Part model, mm, in its own coordinate system. Coordinates: 2 decimals unless noted, no trailing zeros. Loops run counter-clockwise (first coordinate to the right, second up) from the corner with the lowest first, then second, coordinate; pieces in that order, holes last.
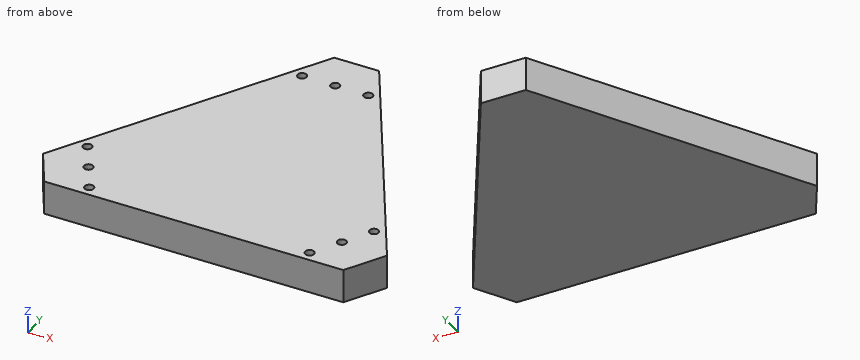
```python
from build123d import *

# Parameters (mm, degrees)
F1_DEPTH = 30
F2_SIZE  = 40
F3_R     = 4
F4_DEPTH = 10


with BuildPart() as f1:
    # F0 (on Top) → F1 (new body)
    with BuildSketch(Plane.XY):
        Polygon((-173.205081, -100), (173.205081, -100), (0, 200), align=None)
    extrude(amount=F1_DEPTH)

    # F2
    f2_edges = [f1.edges().sort_by_distance(p)[0] for p in [
        (-173.205081, -100, 15),
        (173.205081, -100, 15),
        (0, 200, 15),
    ]]
    chamfer(f2_edges, length=F2_SIZE)

    # F3 (on face) → F4 (cut)
    with BuildSketch(Plane.XY.offset(30)):
        with Locations((-29.5, 130.358984)):
            Circle(F3_R)
        with Locations((29.5, 130.358984)):
            Circle(F3_R)
        with Locations((-98.144192, -90.727241)):
            Circle(F3_R)
        with Locations((-127.644192, -39.631743)):
            Circle(F3_R)
        with Locations((127.644192, -39.631743)):
            Circle(F3_R)
        with Locations((98.144192, -90.727241)):
            Circle(F3_R)
        with Locations((0, 130.358984)):
            Circle(F3_R)
        with Locations((-112.894192, -65.179492)):
            Circle(F3_R)
        with Locations((112.894192, -65.179492)):
            Circle(F3_R)
    extrude(amount=-F4_DEPTH, mode=Mode.SUBTRACT)


solid = f1.part
```
Q1. Saw through at C-C (y = -50). List the corners of the cut face in (x, z), plus the area to 3 significant figures.
Q2. Saw through at D-D (x = 66.5). List the corners of the cut face in (y, z), plus the area to 3 significant figures.
Q3. Saw through at B-B (x = -29.5). List the corners of the cut face in (y, z), plus the area to 3 significant figures.
Q4. Saw through at A-A (z = 9). List the corners of the cut face in (x, y), plus the area to 3 significant figures.
Q5. Drop flat-ended pins along their axis: P1, Ø4, axis at y = 30.5, z = 7, coming from the +X side; P2, Ø6.5, axis at x = 112.89, y = -65.18, coming from the +Z side; P3, Ø10, axis at y = 15, z = 22, coming from the -X side; P4, Ø9, axis at x = 31.5, y = 129.5, coming from the +Z side. Give the stop position or say it passes through.
Q6. Probe line 1 (Y direction, x = 126, z = 28); line 2 (X direction, y = 23, z = 12.5); line 3 (Y direction, x = -136.5, z = 23.5). List the from-to ranges inside material, lowest first.
Checked values:
1. outline: (-144.34, 0) - (144.34, 0) - (144.34, 30) - (-144.34, 30) - close
1. area: 8,660 mm2
2. outline: (-100, 0) - (84.82, 0) - (84.82, 30) - (-100, 30) - close
2. area: 5,540 mm2
3. outline: (-100, 0) - (148.9, 0) - (148.9, 30) - (134.36, 30) - (134.36, 20) - (126.36, 20) - (126.36, 30) - (-100, 30) - close
3. area: 7,390 mm2
4. outline: (-153.21, -65.36) - (-133.21, -100) - (133.21, -100) - (153.21, -65.36) - (20, 165.36) - (-20, 165.36) - close
4. area: 49,900 mm2
5. P1: stops at x = 99.02
5. P2: stops at z = 20
5. P3: stops at x = -109.7
5. P4: stops at z = 30
6. line 1: y = -100 to -43.28, -35.99 to -18.24
6. line 2: x = -102.19 to 102.19
6. line 3: y = -94.29 to -36.42
